Print and shaded views of the part. All mm, measured from the part's lowest x, y and z. Coordinates: 2 decimals unless noted, no trailing zeros. Loops run counter-clockwise (first coordinate to the right, second up) from the corner with the lowest first, then second, coordinate; pieces in that order, holes last. Notation, with made-up numbers: M -21,13.5 L -3,13.5 A32 ccw -3,42.5 Z; hole C 67.25,44 d11. An arc over 180 degrees is marked long. Use a Markdown table: item, result. Add a question column.
1) Band-saw the part on A-A (y = 70). State how many separate pieces and enclosed holes the cut face has, plus the area to 3 significant figures.
2) Band-saw the part on D-D (x = 423). List the corners of the cut face in (y, z), plus the area to 3 significant figures.
3) Pin check, flat tip, straight feed: pin 1 Ø1.8 at (x, z) = (420.5, 3.5) entering from +Y. Stop position of the tip, or through.
4) Wall check: probe 1 along X at (y, z) = (53.5, 2.1); probe 2 along Y at (x, z) = (333, 5.45). Give the ranges that are in metal, low to high. Write a range as from..to.
5) Band-saw the part on B-B (y = 45.5). List the corners of the cut face in (x, z).
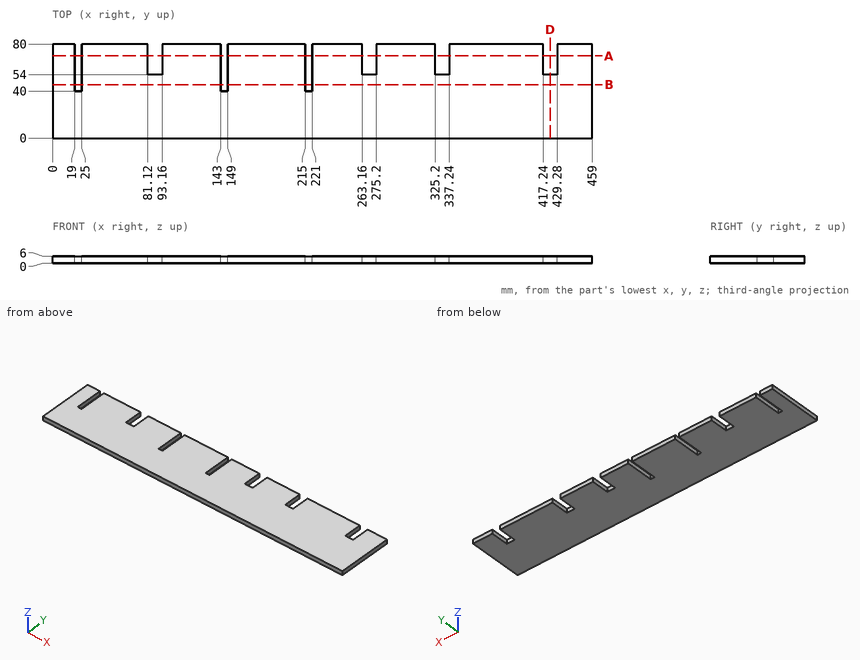
Entries:
| question | item | result |
|---|---|---|
| 1 | separate pieces | 8 |
| 1 | enclosed holes | 0 |
| 1 | area | 2,360 mm2 |
| 2 | outline | M 0,0 L 54,0 L 54,6 L 0,6 Z |
| 2 | area | 324 mm2 |
| 3 | pin 1 | y = 54 |
| 4 | probe 1 | 0..19, 25..143, 149..215, 221..459 |
| 4 | probe 2 | 0..54 |
| 5 | outline | M 0,0 L 19,0 L 19,6 L 0,6 Z; M 25,0 L 143,0 L 143,6 L 25,6 Z; M 149,0 L 215,0 L 215,6 L 149,6 Z; M 221,0 L 459,0 L 459,6 L 221,6 Z |
